Geometry check sheet. Reference: the model listing, model coordinates, mm. Coordinates: 2 decimals unless noted, no trailing zeros. Write each loop counter-clockwise with the first axis right and the second up, starting at its lowest first coordinate (ties: lowest second). Pieces come first, ordered by that corner, then holes. Notation, with made-up numbers: M 70.5,-15.75 L 119.5,-15.75 A15 cw 119.5,6.25 Z; hole C 82,-26 d10. An arc over 180 degrees is marked long. Put each result on its own line as item: value. Start each with the question number.
1) Cross-section at B-B on z = 2.25. Record the cut outline in (x, y), plus the area to 3 significant figures.
2) Scan lines: line 1 along X through (y, z) = (0.75, 3.95); line 2 along Y through (x, z) = (47.5, 2.7); line 3 along X through (y, z) = (2.75, 1.1). Record each from-to range of solid material in increasing order.
3) Mould release check, pull along Y, two halves, no side actions. Record for faces 1 (the cylindrical face through (-54, 0, 2)), 2 (the flat face through (-60, 0, 2)), 3 (the cylindrical face through (41, 0, 2)), 4 (the cylindrical face through (59.43, 9.4, 2.43)): released by +Y, released by -Y, zero draft, split by the parting line, or undercut.
4) Cross-section at A-A on y = -2.5. Record the cut outline in (x, z).
5) Cross-section at C-C on x = 47.5. Record the cut outline in (y, z).
Autodesk Inventor part; units mm, degrees
ref_plane "YZ Plane" through (0, 0, 0) normal (1, 0, 0) x (0, 1, 0)
ref_plane "XZ Plane" through (0, 0, 0) normal (0, 1, 0) x (-1, 0, 0)
ref_plane "XY Plane" through (0, 0, 0) normal (0, 0, 1) x (1, 0, 0)
sketch "Sketch1" plane through (0, 0, 0) normal (0, 0, 1) x (1, 0, 0)
  line L0 (0, 14) -> (0, -14)
  line L1 (-84, 0) -> (84, 0)
  line L2 (-60, 10) -> (60, 10)
  line L3 (60, 10) -> (60, -10)
  line L4 (60, -10) -> (-60, -10)
  line L5 (-60, -10) -> (-60, 10)
  point P0 (0, 0)
  dimension "d0" = 120
  dimension "d1" = 20
extrude "Extrusion1" add sketch "Sketch1" along normal blind 4.8
sketch "Sketch2" plane through (0, 0, 4.8) normal (0, 0, 1) x (1, 0, 0)
  line L0 (-60, -10) -> (60, -10)
  line L1 (60, -10) -> (60, 10)
  line L2 (60, 10) -> (-60, 10)
  line L3 (-60, 10) -> (-60, -10)
  circle A0 centre (-47.5, 0) radius 6.5
  circle A1 centre (47.5, 0) radius 6.5
  line L4 (0, 14) -> (0, -14)
  point P0 (0, 0)
  dimension "d4" = 13
  dimension "d5" = 13
  dimension "d6" = 95
extrude "Extrusion2" cut sketch "Sketch2" against normal through all contours A0 | A1
fillet "Fillet1" radius 2 4 edges at (-60, 10, 2.4) (-60, -10, 2.4) (60, 10, 2.4) (60, -10, 2.4)
properties part number "rodFixer"
Answer key:
1. outline: M -60,-8 A2 ccw -58,-10 L 58,-10 A2 ccw 60,-8 L 60,8 A2 ccw 58,10 L -58,10 A2 ccw -60,8 Z; hole C -47.5,0 d13; hole C 47.5,0 d13
1. area: 2,130 mm²
2. line 1: x = -60 to -53.96, -41.04 to 41.04, 53.96 to 60
2. line 2: y = -10 to -6.5, 6.5 to 10
2. line 3: x = -60 to -53.39, -41.61 to 41.61, 53.39 to 60
3. face 1: undercut
3. face 2: zero draft
3. face 3: undercut
3. face 4: released by +Y
4. outline: M -60,0 L -53.5,0 L -53.5,4.8 L -60,4.8 Z; M -41.5,0 L 41.5,0 L 41.5,4.8 L -41.5,4.8 Z; M 53.5,0 L 60,0 L 60,4.8 L 53.5,4.8 Z
5. outline: M -10,0 L -6.5,0 L -6.5,4.8 L -10,4.8 Z; M 6.5,0 L 10,0 L 10,4.8 L 6.5,4.8 Z
